Can you work these out from the model? Positions are in its coordinate system, mm. Round coordinates to 2 decimals unless told otherwise and drop trailing zeros. Loops run counter-clockwise (first coordinate to the right, second up) from the corner with the lowest first, then second, coordinate; pieces in that order, holes last. Notation, with made-up numbers: (26.25, -31.75) -> (30.25, -31.75) arc R15 cw to (30.25, -12.75) -> close; hole circle Ø1 at (42, -29.75). An arc over 180 degrees is marked (long way). Write item = value, one per line.
from build123d import *
from build123d.topology import SkipClean

# Parameters (mm, degrees)
SKETCH1_R           = 2
BOSS_EXTRUDE1_DEPTH = 76.2
BOSS_EXTRUDE2_DEPTH = 76.2


with BuildPart() as part:
    # Sketch1 → Boss-Extrude1 (new body)
    with BuildSketch(Plane.XY):
        with Locations(Location((0, 0, 0), (0, 0, 180))):
            Circle(SKETCH1_R)
    extrude(amount=BOSS_EXTRUDE1_DEPTH)

    # Sketch2 → Boss-Extrude2 (add)
    with SkipClean():  # the faces are left unmerged after this step: merging them gives an invalid solid
        with BuildSketch(Plane.XY.offset(76.2)):
            with BuildLine():
                Line((-0.79375, 1.835745336), (-0.79375, 1.0475))
                Line((-0.79375, 1.0475), (0.79375, 1.0475))
                Line((0.79375, 1.0475), (0.79375, 1.835745336))
                ThreePointArc((0.79375, 1.835745336), (0, -2), (-0.79375, 1.835745336))
            make_face()
        extrude(amount=BOSS_EXTRUDE2_DEPTH)


solid = part.part
1. Suppose I cut it at A-A, the plane x = 0. List the corners of the cut face in (y, z) for me, and give its area (3 significant figures).
Entries:
outline = (-2, 0) -> (2, 0) -> (2, 76.2) -> (1.05, 76.2) -> (1.05, 152.4) -> (-2, 152.4) -> close
area = 537 mm²
2. I'm going to push flat-ended pins straight in: pin 1 (0.8 mm diameter, centred on x = 0, y = 1.5, fed in from +Z); pin 2 (0.9 mm diameter, centred on y = 1.5, z = 125, fed in from +X); pin 3 (0.5 mm diameter, centred on x = 0.5, z = 96, fed in from +Y). Where does each tip first touch, or does it pass through?
Entries:
pin_1 = 76.2
pin_2 = 1.7
pin_3 = 1.05
3. Suppose I cut it at D-D, the plane z = 115.5. List the corners of the cut face in (x, y) for me.
Entries:
outline = (-0.79, 1.05) -> (-0.79, 1.84) arc R2 ccw (long way) to (0.79, 1.84) -> (0.79, 1.05) -> close
4. Suppose I cut it at C-C, the plane y = -1.2. List the corners of the cut face in (x, z) for me.
Entries:
outline = (-1.6, 0) -> (1.6, 0) -> (1.6, 152.4) -> (-1.6, 152.4) -> close
5. I need wall thicknesses on line 1 (Y direction, x = 0.1, z = 13); line 2 (Z direction, x = -0.7, y = 1.3); line 3 (Y direction, x = -0.15, z = 85). Which ranges of each line are inside material? Lowest first, please. Write a range as [from, to].
Entries:
line_1 = [-2, 2]
line_2 = [0, 76.2]
line_3 = [-1.99, 1.05]
6. Suppose I cut it at B-B, the plane z = 69. List the corners of the cut face in (x, y) for me.
Entries:
outline = circle Ø4 at (0, 0)
